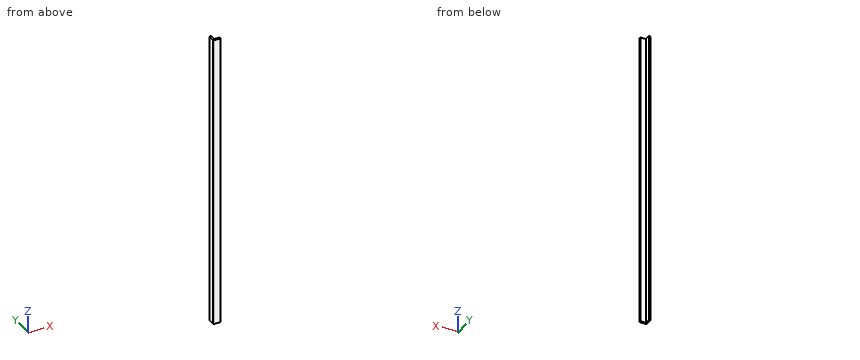
from build123d import *

# Parameters (mm, degrees)
BOSS_EXTRUDE1_DEPTH = 340.5
FILLET1_R           = 1


with BuildPart() as part:
    # Sketch1 → Boss-Extrude1 (new body)
    with BuildSketch(Plane.XY):
        Polygon((0, 0), (-8.5, 0), (-8.5, 8.5), (-6.5, 8.5), (-6.5, 2), (0, 2), align=None)
    extrude(amount=BOSS_EXTRUDE1_DEPTH)

    # Fillet1
    fillet1_edges = [part.edges().sort_by_distance(p)[0] for p in [
        (-8.5, 0, 170.25),
    ]]
    fillet(fillet1_edges, radius=FILLET1_R)


solid = part.part
Check sheet for the modelled part. Datum: model origin and axes. Units: mm. Round coordinates to 2 decimals unless told otherwise and drop trailing zeros. Loops run counter-clockwise (first coordinate to the right, second up) from the corner with the lowest first, then second, coordinate; pieces in that order, holes last. Notation, with made-up numbers: (69, -4.75) - (94, -4.75) arc R16 ccw to (94, 23.25) - close; hole circle Ø3 at (26, -1.5). An arc over 180 degrees is marked (long way). Answer as CSV lines item,"result". Start each with the question number.
Item 1: Section check B-B (y = 3.5). Record the boundary of the cut face in (x, z), and give its area (3 significant figures).
Item 2: Section check A-A (z = 62). Record the boundary of the cut face in (x, y).
Item 3: Scan lines: line 1 (Y direction, x = -3.5, z = 137); line 2 (X direction, y = 4.5, z = 145); line 3 (X direction, y = 0.5, z = 256). Record each from-to range of solid material in increasing order. Write a range as [from, to].
Item 4: Depth check by flat-ended pin: P1, Ø2, axis at x = -1.5, z = 159.5, coming from the +Y side; P2, Ø3, axis at y = 4, z = 224, coming from the +X side. Enter the tip coordinate at first touch or a pass-through.
Item 5: Section check C-C (x = -2.5). Record the boundary of the cut face in (y, z).
Report:
1,outline,"(-8.5, 0) - (-6.5, 0) - (-6.5, 340.5) - (-8.5, 340.5) - close"
1,area,"681 mm2"
2,outline,"(-8.5, 1) arc R1 ccw to (-7.5, 0) - (0, 0) - (0, 2) - (-6.5, 2) - (-6.5, 8.5) - (-8.5, 8.5) - close"
3,line 1,"y = [0, 2]"
3,line 2,"x = [-8.5, -6.5]"
3,line 3,"x = [-8.37, 0]"
4,P1,"stops at y = 2"
4,P2,"stops at x = -6.5"
5,outline,"(0, 0) - (2, 0) - (2, 340.5) - (0, 340.5) - close"
